Check sheet for the modelled part. Datum: model origin and axes. Units: mm. A direction names the side the tool comes from. Coordinates: 2 decimals unless noted, no trailing zeros. Write each loop counter-clockwise with the first axis right and the second up, starting at its lowest first coordinate (ties: lowest second). Pieces come first, ordered by that corner, then holes. Notation, with made-up numbers: M 66.25,-22.75 L 93.25,-22.75 A12 ccw 93.25,-18.75 Z; hole C 36,82 d1. An arc over 180 degrees is marked long. Answer as CSV lines item,"result". Start each with the question number.
1) Material ranges on L1, parallel to X at y = 0.9, z = -47; L2, parallel to Y at x = 49.5, z = -8.5; L3, parallel to X at y = 5.75, z = -7, recorded low to high. Write a range as [from, to].
2) Section check A-A (z = -5). Record the cut outline in (x, y).
3) Section check C-C (y = 4). Record the cut outline in (x, z), and give its area (3 significant figures).
4) Section check D-D (z = -10.5). Record the cut outline in (x, y).
5) Draft check along X on faces 1 (the cylindrical face through (5.07, 1.01, -48.65)), 2 (the flat face through (21, 4, 0)), 3 (the flat face through (56, 1, -26)). Enter one of: +X half, -X half, draft (parallel to the pull), parting line (faces both ways), or undercut.
6) Section check B-B (x = 5). Record the cut outline in (y, z), and give its area (3 significant figures).
7) Access from +Z, -Z, +X, -X, +Y, -Y to the whole of each face (thin tool, end or side, straight path). Record for faces 4 (the flat face through (9.5, 6, -26)), 5 (the flat face through (43, 2, -26)), 6 (the cylindrical face through (52.115, 1.014, -48.216)).
8) Go/stop test with flat-tipped pins: pin 1 Ø6 at (x, z) = (34.5, -28) entering from -Y; pin 2 Ø4 at (y, z) = (6, -18.5) entering from -X; pin 3 Ø2 at (x, z) = (5, -5) entering from -Y; pin 4 Ø13 at (x, z) = (47, -26.5) entering from +Y. Record where each tip stops, or that it passes through.
from build123d import *

# Parameters (mm, degrees)
SKETCH2_W           = 56
SKETCH2_H           = 52
BOSS_EXTRUDE1_DEPTH = 2
SKETCH3_R           = 1.65
CUT_EXTRUDE1_DEPTH  = 77.446059414
SKETCH4_W           = 21
SKETCH4_H           = 52
BOSS_EXTRUDE2_DEPTH = 8


with BuildPart() as part:
    # Sketch2 → Boss-Extrude1 (new body)
    with BuildSketch(Plane(origin=(0, 0, 0), x_dir=(1, 0, 0), z_dir=(0, 1, 0))):
        with Locations((28, 26)):
            Rectangle(SKETCH2_W, SKETCH2_H)
    extrude(amount=BOSS_EXTRUDE1_DEPTH)

    # Sketch3 → Cut-Extrude1 (cut, through all)
    with BuildSketch(Plane(origin=(0, 2, 0), x_dir=(1, 0, 0), z_dir=(0, 1, 0))):
        with Locations(Location((5, 47, 0), (0, 0, 270))):
            Circle(SKETCH3_R)
        with Locations(Location((51, 47, 0), (0, 0, 270))):
            Circle(SKETCH3_R)
        with Locations(Location((5, 5, 0), (0, 0, 270))):
            Circle(SKETCH3_R)
        with Locations(Location((51, 5, 0), (0, 0, 270))):
            Circle(SKETCH3_R)
    extrude(amount=-CUT_EXTRUDE1_DEPTH, mode=Mode.SUBTRACT)

    # Sketch4 → Boss-Extrude2 (add)
    with BuildSketch(Plane(origin=(0, 2, 0), x_dir=(1, 0, 0), z_dir=(0, 1, 0))):
        with Locations((20, 26)):
            Rectangle(SKETCH4_W, SKETCH4_H)
    extrude(amount=BOSS_EXTRUDE2_DEPTH)


solid = part.part
Results found:
1,L1,"x = [0, 3.35], [6.65, 49.35], [52.65, 56]"
1,L2,"y = [0, 2]"
1,L3,"x = [9.5, 30.5]"
2,outline,"M 0,0 L 3.35,0 L 3.35,2 L 0,2 Z; M 6.65,0 L 49.35,0 L 49.35,2 L 30.5,2 L 30.5,10 L 9.5,10 L 9.5,2 L 6.65,2 Z; M 52.65,0 L 56,0 L 56,2 L 52.65,2 Z"
3,outline,"M 9.5,-52 L 30.5,-52 L 30.5,0 L 9.5,0 Z"
3,area,"1,090 mm2"
4,outline,"M 0,0 L 56,0 L 56,2 L 30.5,2 L 30.5,10 L 9.5,10 L 9.5,2 L 0,2 Z"
5,face 1,"undercut"
5,face 2,"draft"
5,face 3,"+X half"
6,outline,"M 0,-52 L 2,-52 L 2,-48.65 L 0,-48.65 Z; M 0,-45.35 L 2,-45.35 L 2,-6.65 L 0,-6.65 Z; M 0,-3.35 L 2,-3.35 L 2,0 L 0,0 Z"
6,area,"90.8 mm2"
7,face 4,"+Z, -Z, -X, +Y"
7,face 5,"+Z, -Z, +X, +Y"
7,face 6,"+Y, -Y"
8,pin 1,"stops at y = 0"
8,pin 2,"stops at x = 9.5"
8,pin 3,"passes through"
8,pin 4,"stops at y = 2"
